```python
from build123d import *

# Parameters (mm, degrees)
SKETCH1_R           = 6.04
BOSS_EXTRUDE1_DEPTH = 18.52
SKETCH2_R           = 2.405
CUT_EXTRUDE1_DEPTH  = 18.52
SKETCH3_R           = 2.915
CUT_EXTRUDE2_DEPTH  = 18.52
CHAMFER1_SIZE       = 0.69
CHAMFER2_SIZE       = 0.69


with BuildPart() as part:
    # Sketch1 → Boss-Extrude1 (new body)
    with BuildSketch(Plane.XY):
        Circle(SKETCH1_R)
    extrude(amount=BOSS_EXTRUDE1_DEPTH)

    # Sketch2 → Cut-Extrude1 (cut)
    with BuildSketch(Plane.XY.offset(18.52)):
        Circle(SKETCH2_R)
    extrude(amount=-CUT_EXTRUDE1_DEPTH, mode=Mode.SUBTRACT)

    # Sketch3 → Cut-Extrude2 (cut)
    with BuildSketch(Plane.XY.offset(18.52)):
        Circle(SKETCH3_R)
    extrude(amount=-CUT_EXTRUDE2_DEPTH, mode=Mode.SUBTRACT)

    # Chamfer1
    chamfer1_edges = [part.edges().sort_by_distance(p)[0] for p in [
        (-2.915, 0, 18.52),
    ]]
    chamfer(chamfer1_edges, length=CHAMFER1_SIZE)

    # Chamfer2
    chamfer2_edges = [part.edges().sort_by_distance(p)[0] for p in [
        (-2.915, 0, 0),
    ]]
    chamfer(chamfer2_edges, length=CHAMFER2_SIZE)


solid = part.part
```
Source: CAD feature listing. Evaluate the final solid. Frame: model axes, mm. Round coordinates to 2 decimals unless told otherwise and drop trailing zeros. Write each loop counter-clockwise with the first axis right and the second up, starting at its lowest first coordinate (ties: lowest second). Pieces come first, ordered by that corner, then holes. Notation, with made-up numbers: M 32,15.5 L 85,15.5 A9 cw 85,22.5 Z; hole C 36,29.5 d9. An arc over 180 degrees is marked long. Answer as a JSON object with one key per item and string values. Group by question number.
(1) Section query C-C on z = 5. Output: boundary loops of the cut face in (x, y) (3 decimals).
(2) Mould query, pull axis X, two halves, no side actions, for faces 1 (the flat face through (3, -3, 18.52)), 2 (the cylindrical face through (2.78, 0.88, 9.38)), 3 (the cylindrical face through (-0.79, 5.99, 9.13)). Classes: +X half, -X half, draft (parallel to the pull), parting line (faces both ways), or undercut.
(3) First-contact query: pin 1 (3 mm diameter, centred on x = -2, y = -0.5, fed in from -Z); pin 2 (2 mm diameter, centred on x = -1, y = -1, fed in from +Z); pin 3 (3 mm diameter, centred on y = -3.5, z = 14.5, fed in from +X). Flat tips, straight axial feed; report the tip coordinate or a pass-through.
(4) Section query A-A on x = 0. Output: boundary loops of the cut face in (y, z) (3 decimals).
(5) Section query D-D on y = -4.25. Output: boundary loops of the cut face in (x, z).
(6) Ray query, line 1 (Y direction, x = 0, z = 10.75) (3 decimals); line 2 (X direction, y = 2, z = 16.5); line 3 (Y direction, x = 1, z = 1.5). Return the intervals inside material, ascending. Write a range as [from, to].
Computed values:
{
 "1": {"outline": "C 0,0 d12.08; hole C 0,0 d5.83"},
 "2": {"face 1": "draft", "face 2": "undercut", "face 3": "parting line"},
 "3": {"pin 1": "z = 0.04", "pin 2": "through", "pin 3": "x = 5.7"},
 "4": {"outline": "M -6.04,0 L -3.605,0 L -2.915,0.69 L -2.915,17.83 L -3.605,18.52 L -6.04,18.52 Z; M 2.915,0.69 L 3.605,0 L 6.04,0 L 6.04,18.52 L 3.605,18.52 L 2.915,17.83 Z"},
 "5": {"outline": "M -4.29,0 L 4.29,0 L 4.29,18.52 L -4.29,18.52 Z"},
 "6": {"line 1": "[-6.04, -2.915], [2.915, 6.04]", "line 2": "[-5.7, -2.12], [2.12, 5.7]", "line 3": "[-5.96, -2.74], [2.74, 5.96]"}
}
